The model under review builds one solid part; all positions refer to its coordinate system, in mm. Face numbers are marked on the shaded views. Round coordinates to 2 decimals unless told otherwise and drop trailing zeros. Write each question's results on one line, items separated by ' | '.
```python
from build123d import *

# Parameters (mm, degrees)
SALIENTE_EXTRUIR1_DEPTH = 2
SALIENTE_EXTRUIR2_START = -2
SALIENTE_EXTRUIR2_DEPTH = 42


with BuildPart() as part:
    # Croquis4 → Saliente-Extruir1 (new body)
    with BuildSketch(Plane(origin=(0, 0, 0), x_dir=(1, 0, 0), z_dir=(0, 1, 0))):
        with BuildLine():
            add(Edge.make_bspline(
                [(52.710297529, 99.582127302), (63.756561517, 138.081595195), (82.710297529, 129.735907435)],
                knots=[0, 0, 0, 0.959481385, 0.959481385, 0.959481385], degree=2))
            add(Edge.make_bspline(
                [(52.710297529, 99.582127302), (90.126545005, 54.518849823), (132.710297529, 59.582127302)],
                knots=[0, 0, 0, 0.796718819, 0.796718819, 0.796718819], degree=2))
            add(Edge.make_bspline(
                [(202.710297529, 109.582127302), (173.420126191, 68.358434503), (132.710297529, 59.582127302)],
                knots=[0, 0, 0, 0.720516106, 0.720516106, 0.720516106], degree=2))
            add(Edge.make_bspline(
                [(194.454170212, 140.507214192), (199.136053193, 125.204121307), (202.710297529, 109.582127302)],
                knots=[0, 0, 0, 0.675598466, 0.675598466, 0.675598466], degree=2))
            add(Edge.make_bspline(
                [(152.449897532, 140.507214192), (182.808256429, 180.784913915), (194.454170212, 140.507214192)],
                knots=[0, 0, 0, 1, 1, 1], degree=2))
            add(Edge.make_bspline(
                [(132.710297529, 119.582127302), (140.11488779, 125.935824124), (146.690299112, 132.884341967), (152.449897532, 140.507214192)],
                knots=[0, 0, 0, 0, 0.833964402, 0.833964402, 0.833964402, 0.833964402], degree=3))
            add(Edge.make_bspline(
                [(102.65877087, 118.201219927), (122.100312055, 109.428474087), (132.710297529, 119.582127302)],
                knots=[0, 0, 0, 0.908986228, 0.908986228, 0.908986228], degree=2))
            add(Edge.make_bspline(
                [(82.710297529, 129.735907435), (92.671997726, 123.923322823), (102.65877087, 118.201219927)],
                knots=[0, 0, 0, 0.910186202, 0.910186202, 0.910186202], degree=2))
        make_face()
    extrude(amount=SALIENTE_EXTRUIR1_DEPTH)


with BuildPart() as saliente_extruir2_tool:
    # Croquis19 → Saliente-Extruir2 (new body)
    with BuildSketch(Plane(origin=(0, 2, 0), x_dir=(1, 0, 0), z_dir=(0, 1, 0)).offset(SALIENTE_EXTRUIR2_START)):
        with BuildLine():
            ThreePointArc((83.62236865, 131.519291558), (93.584161606, 125.732410099), (103.568713537, 119.984885532))
            add(Edge.make_bspline(
                [(131.365719965, 121.063748092), (130.971888683, 120.684835363), (130.142632133, 119.9517928), (128.438784912, 118.697522102), (126.162778494, 117.462528487), (123.183412129, 116.506911998), (119.912471769, 116.071224684), (116.324809268, 116.172759218), (113.063366868, 116.72219656), (110.29220395, 117.449231612), (108.134536322, 118.139339847), (106.268418782, 118.837388441), (104.741437099, 119.467238276), (103.95605498, 119.810793101), (103.568713537, 119.984885532)],
                knots=[0.499479639, 0.499479639, 0.499479639, 0.499479639, 0.499622406, 0.499765174, 0.500050708, 0.500336242, 0.500621776, 0.500907311, 0.501192845, 0.501335612, 0.501478379, 0.501621146, 0.50169253, 0.501763914, 0.501763914, 0.501763914, 0.501763914], degree=3))
            add(Edge.make_bspline(
                [(150.95199089, 141.842528057), (149.526755213, 139.951249583), (146.571479335, 136.248825133), (141.830479534, 130.941084133), (136.787475181, 125.875234297), (133.19424387, 122.632759491), (131.365719965, 121.063748092)],
                knots=[-3.407e-05, -3.407e-05, -3.407e-05, -3.407e-05, 0.210052577, 0.420139224, 0.630225871, 0.840312518, 0.840312518, 0.840312518, 0.840312518], degree=3))
            add(Edge.make_bspline(
                [(196.371161118, 141.077635904), (196.248795755, 141.500563841), (195.995397252, 142.352285229), (195.48073896, 143.986147771), (194.809972536, 145.941130105), (193.963876481, 148.134691236), (192.777490455, 150.861896983), (191.18107336, 153.901083064), (188.359000505, 157.974905621), (184.238162706, 161.603811097), (178.221700824, 163.150703065), (172.92813627, 161.916340062), (168.615333395, 159.654290079), (165.303845353, 157.336157381), (161.897909374, 154.406523973), (158.966988471, 151.456103514), (156.561279242, 148.789333407), (154.72613836, 146.636533397), (153.168453014, 144.712387311), (151.909452091, 143.100825644), (151.267942364, 142.260777118), (150.95199089, 141.842528057)],
                knots=[0.497988609, 0.497988609, 0.497988609, 0.497988609, 0.498059528, 0.498130447, 0.498272286, 0.498414124, 0.498555962, 0.498839638, 0.499123315, 0.499690668, 0.500258021, 0.500825374, 0.50110905, 0.501392727, 0.501676403, 0.501960079, 0.502101918, 0.502243756, 0.502385594, 0.502456513, 0.502527432, 0.502527432, 0.502527432, 0.502527432], degree=3))
            add(Edge.make_bspline(
                [(204.858492638, 109.156288537), (204.249367291, 111.843236182), (202.981172007, 117.207552496), (200.93288469, 125.208306826), (198.73765845, 133.167598608), (197.176202956, 138.445971282), (196.371161118, 141.077635904)],
                knots=[0.499571789, 0.499571789, 0.499571789, 0.499571789, 0.499709653, 0.499847517, 0.499985381, 0.500123245, 0.500123245, 0.500123245, 0.500123245], degree=3))
            add(Edge.make_bspline(
                [(133.039987072, 57.607298121), (136.517017027, 58.353588239), (143.410304061, 60.211208361), (153.331921439, 64.042793156), (162.890265106, 68.929810065), (172.064001952, 74.864194253), (180.854741648, 81.841702982), (187.85941484, 88.520970761), (193.271403672, 94.381452844), (197.234097167, 99.034056041), (200.458372672, 103.128234116), (202.986483638, 106.526999655), (204.241393684, 108.278784185), (204.858492638, 109.156288537)],
                knots=[0.499550345, 0.499550345, 0.499550345, 0.499550345, 0.499920524, 0.500290703, 0.500660881, 0.50103106, 0.501401239, 0.501771418, 0.501956507, 0.502141596, 0.502326686, 0.50241923, 0.502511775, 0.502511775, 0.502511775, 0.502511775], degree=3))
            add(Edge.make_bspline(
                [(50.499998363, 99.117827857), (51.28713851, 98.159265707), (52.890478228, 96.244606437), (56.086666196, 92.579661214), (60.120878243, 88.23562625), (65.006762747, 83.424905696), (71.588596042, 77.539618496), (79.941105501, 71.180357421), (90.169736046, 65.152928032), (100.604072147, 60.742602073), (111.233689738, 57.963400667), (120.24760203, 57.016603306), (127.525650082, 57.079807576), (131.212661015, 57.387753526), (133.039987072, 57.607298121)],
                knots=[0.497081408, 0.497081408, 0.497081408, 0.497081408, 0.49719343, 0.497305453, 0.497529497, 0.497753542, 0.497977587, 0.498425676, 0.498873765, 0.499321855, 0.499769944, 0.500218033, 0.500442078, 0.500666123, 0.500666123, 0.500666123, 0.500666123], degree=3))
            add(Edge.make_bspline(
                [(83.62236865, 131.519291558), (83.190564237, 131.711951172), (82.306221846, 132.074777828), (80.565610632, 132.658261641), (78.390963008, 133.138657799), (75.809004868, 133.290414791), (72.428155416, 132.910719977), (68.40918787, 131.337949061), (64.074405033, 127.853972923), (60.176273009, 122.906250357), (57.22522126, 117.581734073), (55.018923032, 112.59516445), (53.438684901, 108.492028222), (52.179464056, 104.761070862), (51.210491315, 101.605518316), (50.730590106, 99.941775987), (50.499998363, 99.117827857)],
                knots=[0.499165355, 0.499165355, 0.499165355, 0.499165355, 0.49927472, 0.499384085, 0.499602815, 0.499821545, 0.500040276, 0.500477736, 0.500915196, 0.501352656, 0.501790116, 0.502008846, 0.502227576, 0.502446306, 0.502555671, 0.502665036, 0.502665036, 0.502665036, 0.502665036], degree=3))
        make_face()
        with BuildLine():
            ThreePointArc((82.71029754, 129.73590743), (92.673161251, 123.948894915), (102.658770868, 118.201219928))
            add(Edge.make_bspline(
                [(132.710297529, 119.582127302), (122.100312054, 109.428474087), (102.658770868, 118.201219928)],
                knots=[0, 0, 0, 1, 1, 1], degree=2))
            add(Edge.make_bspline(
                [(152.54853475, 140.637933075), (146.765405271, 132.963757867), (140.157191664, 125.972124037), (132.710297529, 119.582127302)],
                knots=[0, 0, 0, 0, 0.838729004, 0.838729004, 0.838729004, 0.838729004], degree=3))
            add(Edge.make_bspline(
                [(194.454170212, 140.507214192), (182.827185257, 180.719448068), (152.54853475, 140.637933075)],
                knots=[0, 0, 0, 1, 1, 1], degree=2))
            add(Edge.make_bspline(
                [(202.710297591, 109.58212739), (199.136053222, 125.204121351), (194.454170212, 140.507214192)],
                knots=[0, 0, 0, 1, 1, 1], degree=2))
            add(Edge.make_bspline(
                [(132.710297645, 59.582127316), (173.420126277, 68.358434565), (202.710297591, 109.58212739)],
                knots=[0, 0, 0, 1, 1, 1], degree=2))
            add(Edge.make_bspline(
                [(52.710297498, 99.582127194), (90.126545043, 54.518849734), (132.710297645, 59.582127316)],
                knots=[0, 0, 0, 1, 1, 1], degree=2))
            add(Edge.make_bspline(
                [(82.71029754, 129.73590743), (63.756561494, 138.081595218), (52.710297498, 99.582127194)],
                knots=[0, 0, 0, 1, 1, 1], degree=2))
        make_face(mode=Mode.SUBTRACT)
    extrude(amount=SALIENTE_EXTRUIR2_DEPTH)


with BuildPart() as part_1:
    add(part.part)


with BuildPart() as part_2:
    # Saliente-Extruir2: joined with saliente_extruir2_tool
    add(part_1.part.fuse(saliente_extruir2_tool.part, tol=0.00001))


solid = part_2.part
```
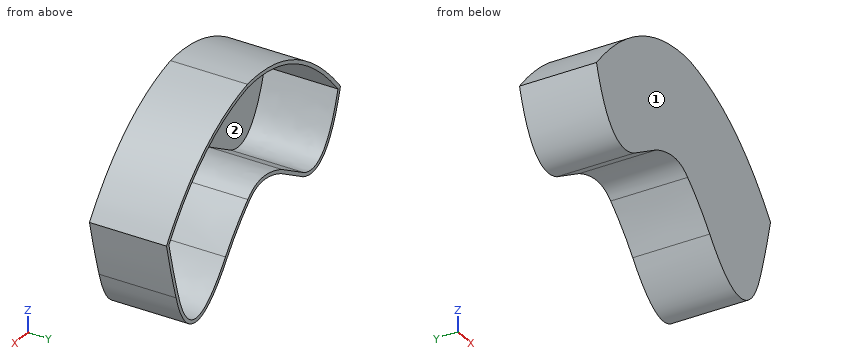
Q1. The part is to be moulded in two halves that separate along X. For the marked faces 1 and 2, say which applies: released by +X, released by -X, zero draft, split by the parting line, or undercut.
Evaluation:
face 1: zero draft | face 2: undercut
Q2. For probe 1 along Z at (x, y) = (113.5, 23); probe 2 along Z at (x, y) = (155, 6); probe 3 along X at (y, z) = (33.5, -66), list the stretches that pass through material, from the lowest coordinate up.
Evaluation:
probe 1: z = -116.68 to -114.65, -59.89 to -57.87 | probe 2: z = -146.95 to -143.79, -67.23 to -65.01 | probe 3: x = 89.08 to 93.6, 152.36 to 157.04
Q3. Insertion check: P1, Ø6, axis at x = 86, y = 22.5, coming from the -Z side; P2, Ø2, axis at x = 70.5, z = -128.5, coming from the +Y side; P3, Ø4, axis at x = 152, y = 23, coming from the -Z side; P4, Ø10, axis at x = 117.5, z = -69, coming from the -Y side. Each pin has a flat end and moves straight along its axis. Give the tip position at first contact, or say it passes through.
Evaluation:
P1: stops at z = -131.79 | P2: stops at y = 2 | P3: stops at z = -145.73 | P4: stops at y = 0
